from build123d import *

# Parameters (mm, degrees)
F0_R       = 38.1
F1_DEPTH   = 12.7
F2_SIZE2   = 10.8824878114
F2_SIZE    = 7.62
F2_2_SIZE2 = 10.8824878114
F2_2_SIZE  = 7.62
F3_R       = 5.08


with BuildPart() as f1:
    # F0 (on Top) → F1 (new body, symmetric)
    with BuildSketch(Plane.XY):
        Circle(F0_R)
    extrude(amount=F1_DEPTH, both=True)

    # F2
    f2_edges = [f1.edges().sort_by_distance(p)[0] for p in [
        (-38.1, 0, 12.7),
    ]]
    f2_side = f1.faces().sort_by_distance((0, 0, 12.7))[0]
    chamfer(f2_edges, length=F2_SIZE, length2=F2_SIZE2, reference=f2_side)

    # F2#2
    f2_2_edges = [f1.edges().sort_by_distance(p)[0] for p in [
        (-38.1, 0, -12.7),
    ]]
    f2_2_side = f1.faces().sort_by_distance((0, 0, -12.7))[0]
    chamfer(f2_2_edges, length=F2_2_SIZE, length2=F2_2_SIZE2, reference=f2_2_side)

    # F3
    f3_edges = [f1.edges().sort_by_distance(p)[0] for p in [
        (-38.1, 0, 1.817512),
        (-30.48, 0, 12.7),
        (-38.1, 0, -1.817512),
        (-30.48, 0, -12.7),
    ]]
    fillet(f3_edges, radius=F3_R)


solid = f1.part
Source: CAD feature listing. Evaluate the final solid. Frame: model axes, mm. Round coordinates to 2 decimals unless told otherwise and drop trailing zeros. Loops run counter-clockwise (first coordinate to the right, second up) from the corner with the lowest first, then second, coordinate; pieces in that order, holes last. Notation, with made-up numbers: (67.25, 55.5) - (118.25, 55.5) arc R29 cw to (118.25, 81.5) - close; hole circle Ø10 at (82, 24). An arc over 180 degrees is marked (long way). Write item = value, one per line. Start each with the question number.
(1) Section query B-B, the plane z = 4.75. Output: boundary loops of the cut face in (x, y), plus the area to 3 significant figures.
(2) Pin query (flat end, axial travel): pin 1 (3 mm diameter, centred on x = 20.5, z = -1, fed in from -Y); pin 2 (10 mm diameter, centred on x = -24.5, z = 1.5, fed in from +Y); pin 3 (8 mm diameter, centred on x = 9.5, z = 1, fed in from +Y). Return the tip coordinate at first contact, or that it passes through.
(3) Ray query, line 1 along X through (y, z) = (18.5, 8.5); line 2 along X through (y, z) = (17, 0.5); line 3 along Y through (x, z) = (17.5, -0.5). Return the intervals inside material, ascending. Write a range as from..to.
(4) Section query A-A, the plane z = -7.75. Output: boundary loops of the cut face in (x, y), plus the area to 3 significant figures.
Conclusion:
q1.outline = circle Ø72.09 at (0, 0)
q1.area = 4,080 mm2
q2.pin_1 = -32.98
q2.pin_2 = 32.67
q2.pin_3 = 37.69
q3.line_1 = -27.83..27.83
q3.line_2 = -34.09..34.09
q3.line_3 = -33.83..33.83
q4.outline = circle Ø67.89 at (0, 0)
q4.area = 3,620 mm2
